Geometry: final body of the model. Coordinates: model frame, mm. Give positions to 0.01 mm unless a question says otherwise; leave off trailing zeros. Write each loop counter-clockwise with the first axis right and the second up, starting at its lowest first coordinate (ties: lowest second). Pieces come first, ordered by that corner, then holes. Notation, with made-up numbers: (17, 51) -> (51, 51) arc R28 ccw to (51, 76) -> close; hole circle Ø6 at (71, -22). An arc over 180 degrees is marked (long way). Answer as a JSON object with one key per item and string values. Group by question number.
(1) Section query B-B on y = 55. Output: boundary loops of the cut face in (x, z), plus the area to 3 significant figures.
(2) Section query A-A on x = -113. Output: boundary loops of the cut face in (y, z), plus the area to 3 significant figures.
(3) Material intervals for probe 1 along Y at (x, z) = (-117, 1.65); probe 2 along Y at (x, z) = (50, 1.9); probe 3 along X at (y, z) = (-56, 4.65), sorted ascending.
from build123d import *

# Parameters (mm, degrees)
ESBO_O1_W                = 430
ESBO_O1_H                = 200
RESSALTO_EXTRUS_O1_DEPTH = 4.7625
CORTE_EXTRUS_O1_DEPTH    = 5.7625


with BuildPart() as part:
    # Esboço1 → Ressalto-extrusão1 (new body)
    with BuildSketch(Plane.XY):
        Rectangle(ESBO_O1_W, ESBO_O1_H)
    extrude(amount=RESSALTO_EXTRUS_O1_DEPTH)

    # Esboço2 → Corte-extrusão1 (cut, through all)
    with BuildSketch(Plane.XY.offset(4.7625)):
        with BuildLine():
            Line((-202.5, 60.5), (-177.5, 60.5))
            ThreePointArc((-177.5, 60.5), (-172, 55), (-177.5, 49.5))
            Line((-177.5, 49.5), (-202.5, 49.5))
            ThreePointArc((-202.5, 49.5), (-208, 55), (-202.5, 60.5))
        make_face()
        with BuildLine():
            Line((-93.5, 49.5), (-118.5, 49.5))
            ThreePointArc((-118.5, 49.5), (-124, 55), (-118.5, 60.5))
            Line((-118.5, 60.5), (-93.5, 60.5))
            ThreePointArc((-93.5, 60.5), (-88, 55), (-93.5, 49.5))
        make_face()
        with BuildLine():
            Line((-202.5, -49.5), (-177.5, -49.5))
            ThreePointArc((-177.5, -49.5), (-172, -55), (-177.5, -60.5))
            Line((-177.5, -60.5), (-202.5, -60.5))
            ThreePointArc((-202.5, -60.5), (-208, -55), (-202.5, -49.5))
        make_face()
        with BuildLine():
            Line((-93.5, -60.5), (-118.5, -60.5))
            ThreePointArc((-118.5, -60.5), (-124, -55), (-118.5, -49.5))
            Line((-118.5, -49.5), (-93.5, -49.5))
            ThreePointArc((-93.5, -49.5), (-88, -55), (-93.5, -60.5))
        make_face()
        with BuildLine():
            Line((49, 44.5), (74, 44.5))
            ThreePointArc((74, 44.5), (79.5, 39), (74, 33.5))
            Line((74, 33.5), (49, 33.5))
            ThreePointArc((49, 33.5), (43.5, 39), (49, 44.5))
        make_face()
        with BuildLine():
            Line((199, 33.5), (174, 33.5))
            ThreePointArc((174, 33.5), (168.5, 39), (174, 44.5))
            Line((174, 44.5), (199, 44.5))
            ThreePointArc((199, 44.5), (204.5, 39), (199, 33.5))
        make_face()
        with BuildLine():
            Line((49, -55.5), (74, -55.5))
            ThreePointArc((74, -55.5), (79.5, -61), (74, -66.5))
            Line((74, -66.5), (49, -66.5))
            ThreePointArc((49, -66.5), (43.5, -61), (49, -55.5))
        make_face()
        with BuildLine():
            Line((199, -66.5), (174, -66.5))
            ThreePointArc((174, -66.5), (168.5, -61), (174, -55.5))
            Line((174, -55.5), (199, -55.5))
            ThreePointArc((199, -55.5), (204.5, -61), (199, -66.5))
        make_face()
    extrude(amount=-CORTE_EXTRUS_O1_DEPTH, mode=Mode.SUBTRACT)


solid = part.part
Answer list:
{
 "1": {"outline": "(-215, 0) -> (-208, 0) -> (-208, 4.76) -> (-215, 4.76) -> close; (-172, 0) -> (-124, 0) -> (-124, 4.76) -> (-172, 4.76) -> close; (-88, 0) -> (215, 0) -> (215, 4.76) -> (-88, 4.76) -> close", "area": "1,700 mm2"},
 "2": {"outline": "(-100, 0) -> (-60.5, 0) -> (-60.5, 4.76) -> (-100, 4.76) -> close; (-49.5, 0) -> (49.5, 0) -> (49.5, 4.76) -> (-49.5, 4.76) -> close; (60.5, 0) -> (100, 0) -> (100, 4.76) -> (60.5, 4.76) -> close", "area": "848 mm2"},
 "3": {"probe 1": "-100 to -60.5, -49.5 to 49.5, 60.5 to 100", "probe 2": "-100 to -66.5, -55.5 to 33.5, 44.5 to 100", "probe 3": "-215 to -207.91, -172.09 to -123.91, -88.09 to 46.71, 76.29 to 171.71, 201.29 to 215"}
}
